Autodesk Inventor part; units mm, degrees
ref_plane "YZ Plane" through (0, 0, 0) normal (1, 0, 0) x (0, 1, 0)
ref_plane "XZ Plane" through (0, 0, 0) normal (0, 1, 0) x (-1, 0, 0)
ref_plane "XY Plane" through (0, 0, 0) normal (0, 0, 1) x (1, 0, 0)
sketch "Sketch1" plane through (0, 0, 0) normal (1, 0, 0) x (0, 1, 0)
  line L0 (-5.8, 12.5) -> (-15, 12.5)
  line L1 (-5.8, -12.5) -> (-15, -12.5)
  line L2 (-5.8, 12.5) -> (8.7, 8.35)
  line L3 (-5.8, -12.5) -> (8.7, -8.35)
  arc A0 (8.7, -8.35) -> (8.7, 8.35) centre (3.8372, 0) ccw
  line L4 (-15, 12.5) -> (-15, 18.5)
  line L5 (-15, 18.5) -> (33.5, 18.5)
  line L6 (33.5, 18.5) -> (33.5, -18.5)
  line L7 (33.5, -18.5) -> (-15, -18.5)
  line L8 (-15, -18.5) -> (-15, -12.5)
  point P0 (0, 0)
  point P1 (-10.4, 12.5)
  point P2 (10.8853, -1.4818)
  point P3 (13.5, 0)
  point P4 (33.5, 0)
  dimension "d0" = 9.2
  dimension "d1" = 25
  dimension "d2" = 12.5
  dimension "d5" = 14.5
  dimension "d6" = 14.5
  dimension "d7" = 9.2
  dimension "d8" = 12.5
  dimension "d9" = 15
  dimension "d10" = 15
  dimension "d11" = 4.15
  dimension "d12" = 4.15
  dimension "d13" = 4.8
  dimension "d14" = 6
  dimension "d15" = 6
  dimension "d16" = 37
  dimension "d29" = 20
extrude "Extrusion1" add sketch "Sketch1" along normal blind 20
sketch "Sketch2" plane through (0, 33.5, 18.5) normal (0, 1, 0) x (1, 0, 0)
  line L0 (0, 31) -> (0, 37)
  line L1 (0, 37) -> (70.5, 37)
  line L2 (70.5, 37) -> (70.5, 0.0995)
  line L3 (70.5, 0.0995) -> (0, 0.0995)
  line L4 (0, 0.0995) -> (0, 37)
  line L5 (20, 37) -> (20, 0)
  point P0 (0, 18.5)
  point P1 (70.5, 18.5498)
  point P2 (0, 31)
  dimension "d19" = 50.5
extrude "Extrusion2" add sketch "Sketch2" along normal blind 10
sketch "Sketch3" plane through (0, 33.5, 18.5) normal (0, -1, 0) x (1, 0, 0)
  line L0 (111, -8.5498) -> (111, -28.5498)
  line L1 (111, -28.5498) -> (70.5, -28.5498)
  line L2 (70.5, -28.5498) -> (70.5, -8.5498)
  line L3 (70.5, -0.0995) -> (70.5, -37)
  line L4 (111, -8.5498) -> (120, -8.5498)
  line L5 (120, -8.5498) -> (120, -37)
  line L6 (120, -37) -> (70.5, -37)
  line L7 (70.5, -37) -> (0, -37)
  line L8 (70.5, -37) -> (59.5, -37)
  line L9 (59.5, -37) -> (59.5, -8.5498)
  line L10 (59.5, -8.5498) -> (70.5, -8.5498)
  point P0 (0, -18.5)
  point P1 (70.5, -18.5498)
  point P2 (70.5, -18.5498)
  point P3 (111, -18.5498)
  dimension "d22" = 20
  dimension "d23" = 20
  dimension "d24" = 0
  dimension "d25" = 40.5
  dimension "d26" = 9
  dimension "d30" = 11
extrude "Extrusion3" add sketch "Sketch3" along normal blind 9.5 and the other way blind 10
sketch "Sketch4" plane through (0, 43.5, 18.5) normal (0, 1, 0) x (1, 0, 0)
  line L0 (111, 8.5498) -> (120, 8.5498)
  line L1 (63, 28.5653) -> (120, 28.5653)
  line L2 (120, 28.5653) -> (120, 8.5498)
  line L3 (120, 8.5498) -> (63, 8.5498)
  line L4 (63, 8.5498) -> (63, 28.5653)
  line L5 (70.5, 0.0995) -> (70.5, 28.5498)
  line L6 (111, 28.5498) -> (111, 8.5498)
  point P0 (0, 18.5)
  point P1 (70.5, 14.3246)
  dimension "d33" = 7.5
  dimension "d34" = 9
extrude "Extrusion4" cut sketch "Sketch4" against normal blind 14.2625
sketch "Sketch5" plane through (0, 43.5, 18.5) normal (0, 1, 0) x (1, 0, 0)
  line L0 (63, 8.5498) -> (63, 28.5653)
  line L1 (63, 8.5498) -> (70.5, 8.5498)
  line L2 (70.5, 8.5498) -> (70.5, -1.0168)
  line L3 (70.5, -1.0168) -> (63, -1.0168)
  line L4 (63, -1.0168) -> (63, 8.5498)
  line L5 (70.5, 0.0995) -> (70.5, 8.5498)
  point P0 (0, 18.5)
  dimension "d47" = 0
extrude "Extrusion5" cut sketch "Sketch5" against normal blind 14.2625
sketch "Sketch7" plane through (59.5, 24, 9.9502) normal (0, 0, 1) x (1, 0, 0)
  line L0 (3.5, 5.2375) -> (3.5, 9.5)
  line L1 (11, 0) -> (11, 5.2375)
  line L2 (3.5, 5.2375) -> (11, 5.2375)
  line L3 (11, 5.2375) -> (11, 0)
  line L4 (11, 0) -> (0, 0)
  line L5 (0, 0) -> (0, 9.5)
  line L6 (0, 9.5) -> (3.5, 9.5)
  line L7 (-39.5, 9.5) -> (3.5, 9.5)
  line L8 (3.5, 9.5) -> (3.5, 19.5)
  point P0 (-59.5, -24)
  dimension "d42" = 11
  dimension "d43" = 0
  dimension "d44" = 0
extrude "Extrusion7" add sketch "Sketch7" along normal blind 8.45
sketch "Sketch8" plane through (63, 43.5, 18.4005) normal (1, 0, 0) x (0, 0, -1)
  line L0 (28.4658, 0) -> (28.4658, -14.2625)
  line L1 (36.9005, 0) -> (0, 0)
  line L2 (28.4658, -9.8625) -> (0, -9.8625)
  line L3 (0, -9.8625) -> (0, 0)
  line L4 (0, 0) -> (28.4658, 0)
  line L5 (28.4658, 0) -> (28.4658, -9.8625)
  line L6 (28.4658, -14.2625) -> (8.4502, -14.2625)
  line L7 (8.4502, -14.2625) -> (8.4502, -19.5)
  line L8 (0, -10) -> (0, 0)
  point P0 (18.4005, -43.5)
  dimension "d48" = 4.4
  dimension "d52" = 0
extrude "Extrusion8" add sketch "Sketch8" along normal blind 7.5
sketch "Sketch9" plane through (0, 43.5, 18.5) normal (0, 1, 0) x (1, 0, 0)
  line L0 (59.5, 37) -> (59.5, 0.0998)
  line L1 (59.5, 0.0998) -> (59.5, 37)
  line L2 (120, 37) -> (120, 8.5498)
  line L3 (59.5, 37) -> (120, 37)
  line L4 (70.5, 28.5653) -> (120, 28.5653)
  line L5 (120, 37) -> (120, 28.5653)
  line L6 (120, 28.5653) -> (70.5, 28.5653)
  line L7 (0, 0.0995) -> (70.5, 0.0995)
  line L8 (70.5, 28.5653) -> (70.5, 0.0995)
  line L9 (70.5, 0.0995) -> (59.5, 0.0998)
  point P0 (0, 18.5)
extrude "Extrusion9" add sketch "Sketch9" along normal blind 16
sketch "Sketch10" plane through (0, 43.5, 18.5) normal (0, 1, 0) x (1, 0, 0)
  line L0 (59.5, 0.0998) -> (59.5, 37)
  line L1 (0, 0.0995) -> (70.5, 0.0995)
  line L2 (59.5, 37) -> (0, 37)
  line L3 (0, 37) -> (0, 0.0995)
  line L4 (0, 0.0995) -> (59.5, 0.0995)
  line L5 (59.5, 0.0995) -> (59.5, 37)
  point P0 (0, 18.5)
  point P1 (59.5, 0.0995)
extrude "Extrusion10" add sketch "Sketch10" along normal blind 16
sketch "Sketch12" plane through (0, 59.5, 18.5) normal (0, 1, 0) x (1, 0, 0)
  line L0 (70.5, 28.5498) -> (70.5, 0.0998)
  line L1 (70.5, 0.0998) -> (0, 0.0998)
  line L2 (0, 0.0998) -> (0, -16.6848)
  line L3 (0, -16.6848) -> (70.5, -16.6848)
  line L4 (70.5, -16.6848) -> (70.5, 0.0998)
  point P0 (0, 18.5)
extrude "Extrusion11" cut sketch "Sketch12" against normal blind 76.325
sketch "Sketch13" plane through (0, 29.2375, 18.5) normal (0, 1, 0) x (1, 0, 0)
  line L0 (111, 8.5498) -> (111, 28.5498)
  line L1 (70.5, 0.0998) -> (70.5, 28.5653)
  line L2 (111, 28.5498) -> (70.5, 28.5498)
  line L3 (70.5, 28.5498) -> (70.5, 28.5653)
  line L4 (70.5, 28.5653) -> (111, 28.5653)
  line L5 (111, 28.5653) -> (111, 28.5498)
  point P0 (0, 18.5)
extrude "Extrusion12" cut sketch "Sketch13" against normal blind 76.325
sketch "Sketch14" plane through (0, 24, 18.5) normal (0, -1, 0) x (1, 0, 0)
  circle A0 centre (115.2, -23.3) radius 2.1
  circle A1 centre (115.2, -13.2) radius 2.1
  line L0 (111, -8.5498) -> (111, -28.5653)
  line L1 (20, -10.15) -> (20, -26.85)
  point P0 (0, -18.5)
  point P1 (20, -18.5)
  dimension "d61" = 4.2
  dimension "d62" = 4.2
  dimension "d63" = 10.1
  dimension "d64" = 4.2
  dimension "d65" = 0
  dimension "d66" = 4.8
extrude "Extrusion13" cut sketch "Sketch14" against normal blind 12.825
pattern_linear "Rectangular Pattern1" count 2 spacing 49 along (-1, 0, 0) of "Extrusion13"
sketch "Sketch15" plane through (0, 24, 18.5) normal (0, -1, 0) x (1, 0, 0)
  line L0 (70.5, -0.0998) -> (70.5, -28.5653)
  line L1 (70.5, -0.0998) -> (120, -0.0998)
  line L2 (120, -0.0998) -> (120, -8.5498)
  line L3 (120, -8.5498) -> (111, -8.5498)
  line L4 (120, -8.5498) -> (111, -8.5498)
  line L5 (111, -8.5498) -> (68.7571, -8.5498)
  line L6 (68.7571, -8.5498) -> (59.5, -8.5498)
  line L7 (59.5, -37) -> (59.5, -0.0998)
  line L8 (59.5, -0.0998) -> (59.5, -8.5498)
  line L9 (59.5, -0.0998) -> (70.5, -0.0998)
  point P0 (0, -18.5)
extrude "Extrusion14" add sketch "Sketch15" against normal blind 35.5
sketch "Sketch16" plane through (120, 24, 18.4002) normal (1, 0, 0) x (0, 0, -1)
  line L0 (7.45, 5.2375) -> (29.4655, 5.2375)
  line L1 (29.4655, 5.2375) -> (29.4655, 38.0522)
  line L2 (29.4655, 38.0522) -> (7.45, 38.0522)
  line L3 (7.45, 38.0522) -> (7.45, 5.2375)
  line L4 (28.4655, 5.2375) -> (8.45, 5.2375)
  line L5 (8.45, 5.2375) -> (8.45, 35.5)
  line L6 (28.4655, 35.5) -> (28.4655, 5.2375)
  point P0 (18.4002, -24)
  dimension "d74" = 0
  dimension "d75" = 1
  dimension "d76" = 1
extrude "Extrusion15" cut sketch "Sketch16" against normal blind 49.6875
properties part number "Holder2"
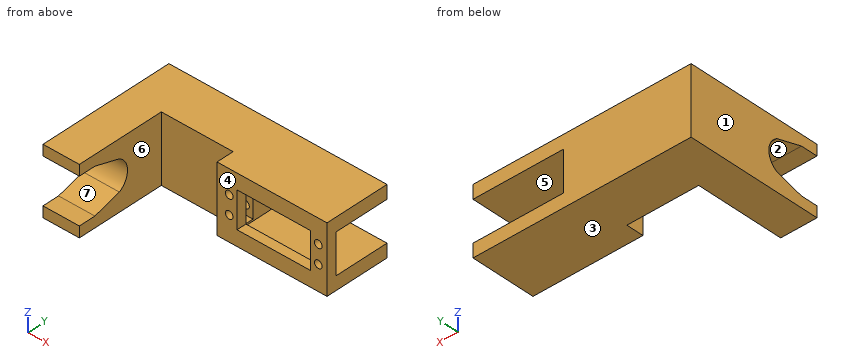
Input: part model. Units: mm. Frame: model coordinates. Face numbers are marked on the shaded views. A direction names the side the tool comes from. Coordinates: 2 decimals unless noted, no trailing zeros. Loops run counter-clockwise (first coordinate to the right, second up) from the corner with the lowest first, then second, coordinate; pieces in that order, holes last.
(1) Pull-direction query (Z, two-part tool) for the marked faces 1, 2 and 3; classes: released by +Z, released by -Z, zero draft, split by the parting line, or undercut.
(2) Section D-D on z = 0.5. Return the cut outline in (x, y).
(3) Set-up query: the marked faces 4, 5, 6 and 7. Return all of +Z, -Z, +X, -X, +Y, -Y with unobstructed straight access to the full face (end or side cutting, diameter ignored); none if empty.
(4) First-contact query: pin 1 Ø6 at (x, z) = (100.5, 6.5) entering from +Y; pin 2 Ø3.5 at (y, z) = (32, 2.5) entering from +X; pin 3 Ø3.5 at (x, z) = (67, -4) entering from -Y; pin 4 Ø4 at (x, z) = (66.2, -4.8) entering from -Y (3 decimals). Flat tips, straight axial feed; report the tip coordinate or a pass-through.
(5) Material intervals for probe 1 along Z at (x, y) = (66.2, 34.8); probe 2 along Z at (x, y) = (98, 51.5); probe 3 along X at (y, z) = (29, 2), sorted ascending.
(6) Section A-A on x = 115.2. Return the cut outline in (y, z).
(7) Section B-B on y = 30.5. Return the cut outline in (x, z).
(8) Section C-C on x = 83.5. Return the cut outline in (y, z).
Data:
1. face 1: zero draft
1. face 2: undercut
1. face 3: released by -Z
2. outline: (0, 13.49) - (20, 13.49) - (20, 33.5) - (59.5, 33.5) - (59.5, 24) - (70.5, 24) - (70.5, 29.24) - (63, 29.24) - (63, 33.64) - (70.31, 33.64) - (70.31, 59.5) - (0, 59.5) - close; (111, 24) - (120, 24) - (120, 29.24) - (111, 29.24) - close
3. face 4: +Z, -Z, +X, -Y
3. face 5: +X, +Y
3. face 6: +Z, -Z, -Y
3. face 7: +X, -X, -Y
4. pin 1: passes through
4. pin 2: stops at x = 70.31
4. pin 3: stops at y = 24
4. pin 4: stops at y = 36.825
5. probe 1: z = -18.5 to -6.9, -2.7 to 3.2, 7.4 to 18.4
5. probe 2: z = -18.5 to -11.07, 10.95 to 18.4
5. probe 3: x = 0 to 20, 59.5 to 70.5, 111 to 120
6. outline: (24, -18.5) - (59.5, -18.5) - (59.5, -11.07) - (29.24, -11.07) - (29.24, -6.9) - (24, -6.9) - close; (24, -2.7) - (29.24, -2.7) - (29.24, 3.2) - (24, 3.2) - close; (24, 7.4) - (29.24, 7.4) - (29.24, 10.95) - (59.5, 10.95) - (59.5, 18.4) - (24, 18.4) - close
7. outline: (0, -18.5) - (20, -18.5) - (20, 18.4) - (0, 18.4) - close; (59.5, -18.5) - (120, -18.5) - (120, -11.07) - (70.31, -11.07) - (70.31, -10.07) - (63, -10.07) - (63, 9.95) - (70.31, 9.95) - (70.31, 10.95) - (120, 10.95) - (120, 18.4) - (59.5, 18.4) - close
8. outline: (24, -18.5) - (59.5, -18.5) - (59.5, -11.07) - (29.24, -11.07) - (29.24, -10.07) - (24, -10.07) - close; (24, 9.95) - (29.24, 9.95) - (29.24, 10.95) - (59.5, 10.95) - (59.5, 18.4) - (24, 18.4) - close
